```python
from build123d import *
from OCP.BRepFilletAPI import BRepFilletAPI_MakeChamfer

# Parameters (mm, degrees)
BOSS_EXTRUDE1_DEPTH        = 93.98
SHELL2_T                   = -5.08
BOSS_EXTRUDE2_DEPTH        = 93.98
SKETCH9_W                  = 31.75
SKETCH9_H                  = 12.7
BOSS_EXTRUDE3_DEPTH        = 25.4
SKETCH8_R                  = 2.1828125
CUT_EXTRUDE2_DEPTH         = 210.869181158
SKETCH10_W                 = 25.4
SKETCH10_H                 = 38.1
BOSS_EXTRUDE4_DEPTH        = 38.1
CHAMFER1_SIZE              = 38.1
CHAMFER1_SIZE_2            = 31.969695948
CHAMFER1_OF_MIRROR3_SIZE   = 38.1
CHAMFER1_OF_MIRROR3_SIZE_2 = 31.969695948
SKETCH13_R                 = 2.1828125
CUT_EXTRUDE4_DEPTH         = 230.473221096
SKETCH15_W                 = 93.98
SKETCH15_H                 = 25.4
CUT_EXTRUDE5_DEPTH         = 230.473221096
CUT_EXTRUDE6_START         = 40.355266
SKETCH14_R                 = 4.191
CUT_EXTRUDE6_DEPTH         = 25.4


with BuildPart() as part:
    # Sketch1 → Boss-Extrude1 (new body)
    with BuildSketch(Plane(origin=(0, 0, 0), x_dir=(0, 0, -1), z_dir=(1, 0, 0))):
        with BuildLine():
            Line((-119.38, 0), (-83.82, 0))
            ThreePointArc((-83.82, 0), (0, -83.82), (83.82, 0))
            Line((83.82, 0), (119.38, 0))
            ThreePointArc((119.38, 0), (0, -119.38), (-119.38, 0))
        make_face()
    extrude(amount=BOSS_EXTRUDE1_DEPTH)

    # Shell2
    shell2_openings = [part.faces().sort_by_distance(p)[0] for p in [
        (46.99, 0, 101.6),
        (46.99, -83.82, 0),
        (46.99, 0, -101.6),
    ]]
    offset(amount=SHELL2_T, openings=shell2_openings, kind=Kind.INTERSECTION)

    # Sketch6 → Boss-Extrude2 (add)
    with BuildSketch(Plane(origin=(0, 0, 0), x_dir=(0, 0, -1), z_dir=(1, 0, 0))):
        with BuildLine():
            Line((-119.38, 0), (-119.38, -119.38))
            Line((-119.38, -119.38), (0, -119.38))
            ThreePointArc((0, -119.38), (-84.414407538, -84.414407538), (-119.38, 0))
        make_face()
    boss_extrude2 = extrude(amount=BOSS_EXTRUDE2_DEPTH)

    # Sketch9 → Boss-Extrude3 (add)
    with BuildSketch(Plane.XY.offset(119.38)):
        with Locations((15.875, -113.03)):
            Rectangle(SKETCH9_W, SKETCH9_H)
        with Locations((78.105, -113.03)):
            Rectangle(SKETCH9_W, SKETCH9_H)
    boss_extrude3 = extrude(amount=BOSS_EXTRUDE3_DEPTH)

    # Sketch8 → Cut-Extrude2 (cut, through all)
    with BuildSketch(Plane(origin=(0, 0, 0), x_dir=(1, 0, 0), z_dir=(0, 1, 0))):
        with Locations(Location((15.875, -132.08, 0), (0, 0, 270))):
            Circle(SKETCH8_R)
        with Locations(Location((78.74, -132.08, 0), (0, 0, 270))):
            Circle(SKETCH8_R)
    cut_extrude2 = extrude(amount=-CUT_EXTRUDE2_DEPTH, mode=Mode.SUBTRACT)

    # Mirror2: Boss-Extrude2, Boss-Extrude3, Cut-Extrude2 across plane
    add(boss_extrude2.mirror(Plane.XY))
    add(boss_extrude3.mirror(Plane.XY))
    add(cut_extrude2.mirror(Plane.XY), mode=Mode.SUBTRACT)

    # Sketch10 → Boss-Extrude4 (add)
    with BuildSketch(Plane.ZY):
        with Locations((-106.68, -100.33)):
            Rectangle(SKETCH10_W, SKETCH10_H)
        with Locations((106.68, -100.33)):
            Rectangle(SKETCH10_W, SKETCH10_H)
    boss_extrude4 = extrude(amount=BOSS_EXTRUDE4_DEPTH)

    # Chamfer1
    chamfer1_edges_1 = [part.edges().sort_by_distance(p)[0] for p in [
        (-38.1, -81.28, 106.68),
    ]]
    chamfer1_side_1 = [part.faces().sort_by_distance(p)[0] for p in [
        (-37.460606081, -81.28, 106.68),
    ]]
    chamfer1_edges_2 = [part.edges().sort_by_distance(p)[0] for p in [
        (-38.1, -81.28, -106.68),
    ]]
    chamfer1_side_2 = [part.faces().sort_by_distance(p)[0] for p in [
        (-37.460606081, -81.28, -106.68),
    ]]
    chamfer1 = BRepFilletAPI_MakeChamfer(part.part.solid().wrapped)
    for e in chamfer1_edges_1:
        chamfer1.Add(CHAMFER1_SIZE - 0.0001, CHAMFER1_SIZE_2 - 0.0001, e.wrapped, chamfer1_side_1[0].wrapped)
    for e in chamfer1_edges_2:
        chamfer1.Add(CHAMFER1_SIZE - 0.0001, CHAMFER1_SIZE_2 - 0.0001, e.wrapped, chamfer1_side_2[0].wrapped)
    add(Compound.cast(chamfer1.Shape()), mode=Mode.REPLACE)  # a hair under: the kernel refuses the full size

    # Mirror3: Boss-Extrude4 across plane
    add(boss_extrude4.mirror(Plane(origin=(46.99, 0, 0), x_dir=(0, 0, 1), z_dir=(1, 0, 0))))

    # Chamfer1 of Mirror3
    chamfer1_of_mirror3_edges_1 = [part.edges().sort_by_distance(p)[0] for p in [
        (132.08, -81.28, 106.68),
    ]]
    chamfer1_of_mirror3_side_1 = [part.faces().sort_by_distance(p)[0] for p in [
        (131.440606081, -81.28, 106.68),
    ]]
    chamfer1_of_mirror3_edges_2 = [part.edges().sort_by_distance(p)[0] for p in [
        (132.08, -81.28, -106.68),
    ]]
    chamfer1_of_mirror3_side_2 = [part.faces().sort_by_distance(p)[0] for p in [
        (131.440606081, -81.28, -106.68),
    ]]
    chamfer1_of_mirror3 = BRepFilletAPI_MakeChamfer(part.part.solid().wrapped)
    for e in chamfer1_of_mirror3_edges_1:
        chamfer1_of_mirror3.Add(CHAMFER1_OF_MIRROR3_SIZE - 0.0001, CHAMFER1_OF_MIRROR3_SIZE_2 - 0.0001, e.wrapped, chamfer1_of_mirror3_side_1[0].wrapped)
    for e in chamfer1_of_mirror3_edges_2:
        chamfer1_of_mirror3.Add(CHAMFER1_OF_MIRROR3_SIZE - 0.0001, CHAMFER1_OF_MIRROR3_SIZE_2 - 0.0001, e.wrapped, chamfer1_of_mirror3_side_2[0].wrapped)
    add(Compound.cast(chamfer1_of_mirror3.Shape()), mode=Mode.REPLACE)  # a hair under: the kernel refuses the full size

    # Sketch13 → Cut-Extrude4 (cut, through all)
    with BuildSketch(Plane(origin=(0, -119.38, 0), x_dir=(1, 0, 0), z_dir=(0, 1, 0))):
        with Locations(Location((-25.4, -106.68, 0), (0, 0, 180))):
            Circle(SKETCH13_R)
        with Locations((119.38, -106.68)):
            Circle(SKETCH13_R)
        with Locations((119.38, 106.68)):
            Circle(SKETCH13_R)
        with Locations(Location((-25.4, 106.68, 0), (0, 0, 180))):
            Circle(SKETCH13_R)
    extrude(amount=CUT_EXTRUDE4_DEPTH, mode=Mode.SUBTRACT)

    # Sketch15 → Cut-Extrude5 (cut, through all)
    with BuildSketch(Plane(origin=(0, -119.38, 0), x_dir=(1, 0, 0), z_dir=(0, 1, 0))):
        with Locations((46.99, -132.08)):
            Rectangle(SKETCH15_W, SKETCH15_H)
        with Locations((46.99, 132.08)):
            Rectangle(SKETCH15_W, SKETCH15_H)
    extrude(amount=CUT_EXTRUDE5_DEPTH, mode=Mode.SUBTRACT)

    # Sketch14 → Cut-Extrude6 (cut)
    with BuildSketch(Plane(origin=(0, -119.38, 0), x_dir=(1, 0, 0), z_dir=(0, 1, 0)).offset(CUT_EXTRUDE6_START)):
        with Locations((-25.4, -106.68)):
            Circle(SKETCH14_R)
        with Locations((119.38, -106.68)):
            Circle(SKETCH14_R)
        with Locations((119.38, 106.68)):
            Circle(SKETCH14_R)
        with Locations((-25.4, 106.68)):
            Circle(SKETCH14_R)
    extrude(amount=-CUT_EXTRUDE6_DEPTH, mode=Mode.SUBTRACT)


solid = part.part
```
Geometry: final body of the model. Coordinates: model frame, mm. A direction names the side the tool comes from. Give positions to 0.01 mm unless a question says otherwise; leave off trailing zeros. Loops run counter-clockwise (first coordinate to the right, second up) from the corner with the lowest first, then second, coordinate; pieces in that order, holes last. Notation, with made-up numbers: (87.5, 58.25) -> (116.5, 58.25) arc R14 ccw to (116.5, 74.25) -> close; hole circle Ø6 at (-8.5, 80.25). An arc over 180 degrees is marked (long way). Use CSV: the item, a comma, the result in double quotes.
(1) Pull-direction query (X, two-part tool) for faces 1 (the face through (43, 0, -115)), 2 (the face through (5.08, -94, -2)), 3 (the face through (113.3, -97.49, 106.5)); classes: released by +X, released by -X, zero draft, split by the parting line, or undercut.
From the geometry:
face 1,"zero draft"
face 2,"undercut"
face 3,"released by +X"
(2) Cut plane A-A (x = -17). Output: boundary loops of the cut face in (y, z).
From the geometry:
outline,"(-119.38, -119.38) -> (-95.54, -119.38) -> (-95.54, -93.98) -> (-119.38, -93.98) -> close; (-119.38, 93.98) -> (-95.54, 93.98) -> (-95.54, 119.38) -> (-119.38, 119.38) -> close"
(3) Access query for faces 4 (the face through (-15, -105, -93.98)), 5 (the face through (46.403, -114.272, -2.513)). Directions: +Z, -Z, +X, -X, +Y, -Y. A direction counts if a zero-diameter tool reaches every point of the face in a straight line with its end or side. Return the directions, or none.
From the geometry:
face 4,"-X, +Y, -Y"
face 5,"+Y"
(4) Cut plane B-B (y = -60). Output: boundary loops of the cut face in (x, z).
From the geometry:
outline,"(0, -119.38) -> (93.98, -119.38) -> (93.98, -58.53) -> (88.9, -58.53) -> (88.9, -97.29) -> (5.08, -97.29) -> (5.08, -58.53) -> (0, -58.53) -> close; (0, 58.53) -> (5.08, 58.53) -> (5.08, 97.29) -> (88.9, 97.29) -> (88.9, 58.53) -> (93.98, 58.53) -> (93.98, 119.38) -> (0, 119.38) -> close"
(5) Cut plane D-D (z = -89.5). Output: boundary loops of the cut face in (x, y).
From the geometry:
outline,"(0, -119.38) -> (93.98, -119.38) -> (93.98, 0) -> (88.9, 0) -> (88.9, -71.09) -> (5.08, -71.09) -> (5.08, 0) -> (0, 0) -> close"
(6) Cut plane C-C (y = -109.5). Output: boundary loops of the cut face in (x, z), plus the area to 3 significant figures.
From the geometry:
outline,"(-33.63, -119.38) -> (127.61, -119.38) -> (127.61, -93.98) -> (93.98, -93.98) -> (93.98, 93.98) -> (127.61, 93.98) -> (127.61, 119.38) -> (-33.63, 119.38) -> (-33.63, 93.98) -> (0, 93.98) -> (0, -93.98) -> (-33.63, -93.98) -> close; hole circle Ø4.37 at (-25.4, -106.68); hole circle Ø4.37 at (-25.4, 106.68); hole (5.08, -32.78) -> (88.9, -32.78) -> (88.9, 32.78) -> (5.08, 32.78) -> close; hole circle Ø4.37 at (119.38, -106.68); hole circle Ø4.37 at (119.38, 106.68)"
area,"20,300 mm^2"
(7) First-contact query: P1, Ø1.9, axis at x = 118, z = -105.5, coming from the +Y side; P2, Ø8, axis at y = -90, z = -86.5, coming from the -X side; P3, Ø2, axis at x = 54, z = -20.5, coming from the +Y side. Flat tips, straight axial feed; report the tip coordinate or a pass-through.
From the geometry:
P1,"y = -104.42"
P2,"x = 0"
P3,"y = -112.26"
(8) Ray query, line 1 along X through (y, z) = (-114.25, 106.68); line 2 along Z through (x, y) = (119.38, -109.25); line 3 along X through (y, z) = (-81.5, 73). Return the intervals inside material, ascending. Write a range as [from, to].
From the geometry:
line 1,"[-38.1, -27.58], [-23.22, 117.2], [121.56, 132.08]"
line 2,"[-119.38, -108.86], [-104.5, -93.98], [93.98, 104.5], [108.86, 119.38]"
line 3,"[0, 5.08], [88.9, 93.98]"
